from build123d import *

# Parameters (mm, degrees)
CROQUIS4_W                   = 38
CROQUIS4_H                   = 2
SALIENTE_EXTRUIR1_DEPTH      = 6
SALIENTE_EXTRUIR1_DEPTH_BACK = 6
CROQUIS1_W                   = 10
CROQUIS1_H                   = 2.5
CORTAR_EXTRUIR2_DEPTH        = 10
CROQUIS5_W                   = 17
CROQUIS5_H                   = 12
CROQUIS5_W_2                 = 10
CORTAR_EXTRUIR3_DEPTH        = 0.2
REDONDEO1_R                  = 0.5
REDONDEO2_R                  = 0.5
REDONDEO4_R                  = 1
CHAFL_N1_SIZE                = 1.5
CHAFL_N1_SIZE2               = 2.598076211
CHAFL_N1_PART_2_SIZE         = 1.5
CHAFL_N1_PART_2_SIZE2        = 2.598076211
REDONDEO5_R                  = 0.5


with BuildPart() as part:
    # Croquis4 → Saliente-Extruir1 (new body, two sides)
    with BuildSketch(Plane(origin=(0, 0, 0), x_dir=(1, 0, 0), z_dir=(0, 1, 0))) as saliente_extruir1_sk:
        with Locations((19, 1)):
            Rectangle(CROQUIS4_W, CROQUIS4_H)
    extrude(amount=SALIENTE_EXTRUIR1_DEPTH)
    extrude(saliente_extruir1_sk.sketch, amount=-SALIENTE_EXTRUIR1_DEPTH_BACK)

    # Croquis1 → Cortar-Extruir2 (cut)
    with BuildSketch(Plane.XY):
        with Locations((33, 4.75)):
            Rectangle(CROQUIS1_W, CROQUIS1_H)
        with Locations((33, -4.75)):
            Rectangle(CROQUIS1_W, CROQUIS1_H)
        with BuildLine():
            Line((5.25, -1), (5.25, 1))
            ThreePointArc((5.25, 1), (3.5, 2.75), (1.75, 1))
            Line((1.75, 1), (1.75, -1))
            ThreePointArc((1.75, -1), (3.5, -2.75), (5.25, -1))
        make_face()
        with BuildLine():
            Line((22.75, 1), (22.75, -1))
            ThreePointArc((22.75, -1), (24.5, -2.75), (26.25, -1))
            Line((26.25, -1), (26.25, 1))
            ThreePointArc((26.25, 1), (24.5, 2.75), (22.75, 1))
        make_face()
    extrude(amount=-CORTAR_EXTRUIR2_DEPTH, mode=Mode.SUBTRACT)

    # Croquis5 → Cortar-Extruir3 (cut)
    with BuildSketch(Plane.XY):
        with Locations((14, 0)):
            Rectangle(CROQUIS5_W, CROQUIS5_H)
        with Locations((33, 0)):
            Rectangle(CROQUIS5_W_2, CROQUIS5_H)
    extrude(amount=-CORTAR_EXTRUIR3_DEPTH, mode=Mode.SUBTRACT)

    # Redondeo1
    redondeo1_edges = [part.edges().sort_by_distance(p)[0] for p in [
        (28, 3.5, -1.1),
        (28, -3.5, -1.1),
    ]]
    fillet(redondeo1_edges, radius=REDONDEO1_R)

    # Redondeo2
    redondeo2_edges = [part.edges().sort_by_distance(p)[0] for p in [
        (22.5, 6, -0.1),
        (22.5, -6, -0.1),
        (5.5, -6, -0.1),
        (5.5, 6, -0.1),
    ]]
    fillet(redondeo2_edges, radius=REDONDEO2_R)

    # Redondeo4
    redondeo4_edges = [part.edges().sort_by_distance(p)[0] for p in [
        (38, 3.5, -1.1),
        (38, -3.5, -1.1),
    ]]
    fillet(redondeo4_edges, radius=REDONDEO4_R)

    # Chaflán1
    chafl_n1_edges = [part.edges().sort_by_distance(p)[0] for p in [
        (0, -6, -1),
        (0, 6, -1),
    ]]
    chafl_n1_side = [part.faces().sort_by_distance(p)[0] for p in [
        (0, 0, -1),
    ]]
    chamfer(chafl_n1_edges, length=CHAFL_N1_SIZE, length2=CHAFL_N1_SIZE2, reference=chafl_n1_side[0])

    # Chaflán1 part 2
    chafl_n1_part_2_edges = [part.edges().sort_by_distance(p)[0] for p in [
        (28, 6, -1),
        (28, -6, -1),
    ]]
    chafl_n1_part_2_side = [part.faces().sort_by_distance(p)[0] for p in [
        (28, 5, -1.878344749),
    ]]
    chamfer(chafl_n1_part_2_edges, length=CHAFL_N1_PART_2_SIZE, length2=CHAFL_N1_PART_2_SIZE2, reference=chafl_n1_part_2_side[0])

    # Redondeo5
    redondeo5_edges = [part.edges().sort_by_distance(p)[0] for p in [
        (25.401923789, 6, -1),
        (2.598076211, 6, -1),
        (0, -4.5, -1),
        (0, 4.5, -1),
        (25.401923789, -6, -1),
        (2.598076211, -6, -1),
        (28, -4.5, -1),
        (28, 4.5, -1),
    ]]
    fillet(redondeo5_edges, radius=REDONDEO5_R)


solid = part.part
Build history of the part. All positions in model axes, mm. A direction names the side the tool comes from. Give positions to 0.01 mm unless a question says otherwise; leave off trailing zeros. Loops run counter-clockwise (first coordinate to the right, second up) from the corner with the lowest first, then second, coordinate; pieces in that order, holes last. Notation, with made-up numbers: (86, 21.25) - (100, 21.25) arc R24 ccw to (100, 54.25) - close; hole circle Ø7 at (3, -21.75). An arc over 180 degrees is marked (long way). Write item = value, one per line. Start each with the question number.
1) Band-saw the part on D-D on x = 9. Give the cut face in (y, z), plus the area to 3 significant figures.
2) Probe probe 1 along X at (y, z) = (0, -1.25); probe 2 along X at (y, z) = (-1, -0.1); probe 3 along X at (y, z) = (-1.75, -0.5). List the from-to ranges inside material, lowest first. Write a range as from..to.
3) Pull direction X, two halves, no side cores. Call faces 1 (the cylindrical face through (3.46, -2.75, -0.99)), 2 (the flat face through (26.618, 5.298, -0.986)), 3 (the cylindrical face through (24.54, 2.75, -0.99)), 4 (the flat face through (33, 3.5, -1)): +X half, -X half, draft (parallel to the pull), parting line (faces both ways), or undercut.
4) Band-saw the part on B-B on y = -0.25. Give the cut face in (x, z).
5) Band-saw the part on A-A on x = 24.5. Give the cut face in (y, z), plus the area to 3 significant figures.
6) Tool access for faces 5 (the flat face through (33, -3.5, -1)), 6 (the flat face through (5.25, 0, -1)), 7 (the flat face through (1.382, -5.298, -0.986)): list every direction of +Z, -Z, +X, -X, +Y, -Y with a clear straight run to the whole face (end or side of a thin tool).
7) Band-saw the part on C-C on z = -0.9. Count the separate pieces of the cut face and the enclosed holes in it, plus the area to 3 significant figures.
8) Drop flat-ended pins along their axis: pin 1 Ø0.9 at (x, z) = (32.5, -0.5) entering from +Y; pin 2 Ø1 at (x, y) = (14, 2) entering from +Z. Give the stop position or say it passes through.
Final values:
q1.outline = (-6, -2) - (6, -2) - (6, -0.2) - (-6, -0.2) - close
q1.area = 21.6 mm²
q2.probe_1 = 0..1.75, 5.25..22.75, 26.25..38
q2.probe_2 = 0..1.75, 5.25..5.5, 22.5..22.75, 26.25..28
q2.probe_3 = 0..1.92, 5.08..22.92, 26.08..38
q3.face_1 = undercut
q3.face_2 = +X half
q3.face_3 = undercut
q3.face_4 = draft
q4.outline = (0, -2) - (1.75, -2) - (1.75, 0) - (0, 0) - close; (5.25, -2) - (22.75, -2) - (22.75, 0) - (22.5, 0) - (22.5, -0.2) - (5.5, -0.2) - (5.5, 0) - (5.25, 0) - close; (26.25, -2) - (38, -2) - (38, -0.2) - (28, -0.2) - (28, 0) - (26.25, 0) - close
q5.outline = (-6, -2) - (-2.75, -2) - (-2.75, 0) - (-6, 0) - close; (2.75, -2) - (6, -2) - (6, 0) - (2.75, 0) - close
q5.area = 13.0 mm²
q6.face_5 = +Z, -Z, +X, -Y
q6.face_6 = +Z, -Z
q6.face_7 = +Z, -Z, -X, -Y
q7.separate_pieces = 1
q7.enclosed_holes = 2
q7.area = 365 mm²
q8.pin_1 = 3.5
q8.pin_2 = -0.2
